Read the model definition and answer for the solid it produces. Units are mm, in the model's axes. A direction names the side the tool comes from. Round coordinates to 2 decimals unless told otherwise and drop trailing zeros. Write each loop counter-clockwise with the first axis right and the second up, starting at its lowest first coordinate (ties: lowest second). Pieces come first, ordered by that corner, then holes. Notation, with made-up numbers: (88, -20.75) - (115, -20.75) arc R23 ccw to (115, 9.25) - close; hole circle Ø5 at (61.5, 89). An arc over 180 degrees is marked (long way). Use one line per item in the form item = value. Start each with the question number.
1) For faces 4 (the face through (-8, 0, -10)), 5 (the face through (47.66, 3, -0.46)), 6 (the face through (81, 0, -4)), determine the directions among +Z, -Z, +X, -X, +Y, -Y from which every point of the face is accessible in a straight line to the end or side of a thin tool.
2) Consider line 1 along X through (y, z) = (-2, -3.5); line 2 along X through (y, z) = (8.5, -16); line 3 along Y through (x, z) = (11, -10.5). Determine where each line is inside the solid, lowest interval first. Write a range as from..to.
3) Each of these flat-tipped pins is pushed along its axis until it touches: pin 1 (1 mm diameter, centred on x = 7.5, z = -2, fed in from +Y); pin 2 (5 mm diameter, centred on x = 68, z = -20, fed in from -Y); pin 3 (3 mm diameter, centred on y = 2.5, z = 0, fed in from +X). Where does it stop, or does it pass through?
4) The part is cut by section C-C, the plane x = 28. Give the vertices of the cut face in (y, z).
5) The part is cut by section A-A, the plane y = 0. Give the vertices of the cut face in (x, z), plus the area to 3 significant figures.
6) For a pull along X with two mould halves and no side action, classify faces 1 (the face through (-1.97, -15.62, -13.47)), 2 (the face through (80, 0, -2)), 3 (the face through (-7.7, -12, -12.7)) as released by +X, released by -X, zero draft, split by the parting line, or undercut.
7) The part is cut by section B-B, the plane z = -10. Give the vertices of the cut face in (x, y).
from build123d import *

# Parameters (mm, degrees)
CUT_EXTRUDE2_DEPTH      = 1
CUT_EXTRUDE2_DEPTH_BACK = 57


with BuildPart() as part:
    # Sketch1 → Revolve1 (revolve)
    with BuildSketch(Plane(origin=(0, 0, 0), x_dir=(1, 0, 0), z_dir=(0, 1, 0))):
        Polygon((0, 0), (94, 0), (96, 2), (96, 10), (-8, 10), (-8, -2), (-4, -6), (0, -6), align=None)
    revolve(axis=Axis((67.877257865, 0, -10), (-1, 0, 0)))

    # Sketch2 → Cut-Extrude2 (cut, two sides)
    with BuildSketch(Plane(origin=(0, 40, 0), x_dir=(1, 0, 0), z_dir=(0, 1, 0))) as cut_extrude2_sk:
        Polygon((80, -199.282857121), (80, 0), (80, 4), (83, 4), (83, 0), (83, -199.282857121), (83, -597.848571364), (80, -597.848571364), align=None)
    extrude(amount=CUT_EXTRUDE2_DEPTH, mode=Mode.SUBTRACT)
    extrude(cut_extrude2_sk.sketch, amount=-CUT_EXTRUDE2_DEPTH_BACK, mode=Mode.SUBTRACT)


solid = part.part
Geometry results:
q1.face_4 = +Z, -Z, -X, +Y, -Y
q1.face_5 = +X
q1.face_6 = +Z, +Y, -Y
q2.line_1 = -8..80, 83..96
q2.line_2 = -8..0
q2.line_3 = -9.99..9.99
q3.pin_1 = 6.61
q3.pin_2 = -6.61
q3.pin_3 = 95.19
q4.outline = circle Ø20 at (0, -10)
q5.outline = (-8, -22) - (-4, -26) - (0, -26) - (0, -20) - (94, -20) - (96, -18) - (96, -2) - (94, 0) - (83, 0) - (83, -4) - (80, -4) - (80, 0) - (0, 0) - (0, 6) - (-4, 6) - (-8, 2) - close
q5.area = 2,140 mm2
q6.face_1 = zero draft
q6.face_2 = undercut
q6.face_3 = released by -X
q7.outline = (-8, -12) - (-4, -16) - (0, -16) - (0, -10) - (94, -10) - (96, -8) - (96, 8) - (94, 10) - (0, 10) - (0, 16) - (-4, 16) - (-8, 12) - close
